Could you check a few things on this model? Use its own coordinates, in mm. Face numbers are marked on the shaded views. Round coordinates to 2 decimals unless told otherwise and drop trailing zeros. Write each loop counter-clockwise with the first axis right and the second up, starting at its lowest first coordinate (ties: lowest second). Pieces come first, ordered by that corner, then holes. Notation, with made-up numbers: (19, 85) -> (51, 85) arc R12 ccw to (51, 92) -> close; hole circle Ø11 at (51, 1). An arc over 180 degrees is marked (long way). Answer in a Markdown table with one row per item.
from build123d import *

# Parameters (mm, degrees)
SKETCH1_W           = 50
SKETCH1_H           = 50
BOSS_EXTRUDE1_DEPTH = 6
CUT_EXTRUDE1_REACH  = 39.336
SKETCH5_R           = 5
CHAMFER1_SIZE       = 1
CHAMFER2_SIZE       = 0.5
M6_TAPPED_HOLE1_D   = 5
SKETCH10_R          = 6.25
CUT_EXTRUDE2_DEPTH  = 2
CIRPATTERN1_COUNT   = 4


# Read off the part's stored shape, not the designer's step: Draft1
with BuildPart() as part:
    # Sketch1 → Boss-Extrude1 (new, symmetric)
    with BuildSketch(Plane.XY):
        Rectangle(SKETCH1_W, SKETCH1_H)
    extrude(amount=BOSS_EXTRUDE1_DEPTH, both=True)

    # Sketch5 → Cut-Extrude1 (cut, up to next)
    with BuildSketch(Plane.XY.offset(6), mode=Mode.PRIVATE) as cut_extrude1_sk1:
        Circle(SKETCH5_R)
    cut_extrude1_tool1 = extrude(cut_extrude1_sk1.sketch, amount=-CUT_EXTRUDE1_REACH, mode=Mode.PRIVATE) & part.part
    add(cut_extrude1_tool1.solids().sort_by_distance((0, 0, 6))[0], mode=Mode.SUBTRACT)

    # Chamfer1
    chamfer1_edges = [part.edges().sort_by_distance(p)[0] for p in [
        (25, -25, 0),
        (-25, -25, 0),
        (-25, 25, 0),
        (25, 25, 0),
    ]]
    chamfer(chamfer1_edges, length=CHAMFER1_SIZE)

    # Chamfer2
    chamfer2_edges = [part.edges().sort_by_distance(p)[0] for p in [
        (0, -25, 6),
        (0, -25, -6),
        (0, 25, -6),
        (0, 25, 6),
        (25, 0, -6),
        (25, 0, 6),
        (-25, 0, -6),
        (-25, 0, 6),
    ]]
    chamfer(chamfer2_edges, length=CHAMFER2_SIZE - 0.0001)  # a hair under: the kernel refuses the full size

    # M6 Tapped Hole1 (through all)
    with Locations(Plane.XY.offset(6)):
        with Locations((-16.5, 0), (0, 16.5), (16.5, 0), (0, -16.5)):
            Hole(M6_TAPPED_HOLE1_D / 2)

    # Sketch10 → Cut-Extrude2 (cut)
    with BuildSketch(Plane.XY.offset(6)):
        with Locations((0, 16.5)):
            Circle(SKETCH10_R)
    cut_extrude2 = extrude(amount=-CUT_EXTRUDE2_DEPTH, mode=Mode.SUBTRACT)

    # CirPattern1: Cut-Extrude2 ×4 about axis
    cirpattern1_axis = Axis((0, 0, 0), (0, 0, 1))
    for i in range(1, CIRPATTERN1_COUNT):
        add(cut_extrude2.rotate(cirpattern1_axis, i * 360 / CIRPATTERN1_COUNT), mode=Mode.SUBTRACT)

    # Draft1 outline → Draft1 (revolve, cut)
    with BuildSketch(Plane.XZ):
        Polygon((5, 6), (5, -2.8), (5.69257502, 6), align=None)
    revolve(axis=Axis((0, 0, 0), (0, 0, 1)), mode=Mode.SUBTRACT)


solid = part.part
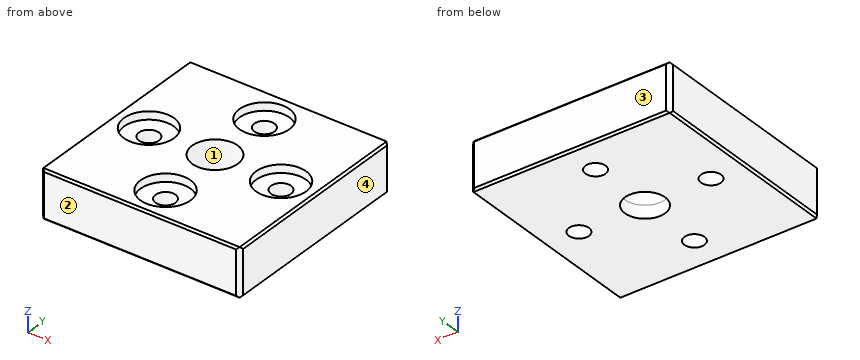
1) Imagine slicing it at D-D, the plane x = 0. Count the separate pieces of the cut face and the enclosed holes in it, plus the area to 3 significant figures.
Findings:
| item | result |
|---|---|
| separate pieces | 4 |
| enclosed holes | 0 |
| area | 323 mm^2 |
2) Imagine slicing it at A-A, the plane x = 16.5. Please give me the cut outline in (y, z), plus the area to 4 significant figures.
Findings:
| item | result |
|---|---|
| outline | (-25, -5.5) -> (-24.5, -6) -> (-2.5, -6) -> (-2.5, 4) -> (-6.25, 4) -> (-6.25, 6) -> (-24.5, 6) -> (-25, 5.5) -> close; (2.5, -6) -> (24.5, -6) -> (25, -5.5) -> (25, 5.5) -> (24.5, 6) -> (6.25, 6) -> (6.25, 4) -> (2.5, 4) -> close |
| area | 524.5 mm^2 |
3) For pin 1 (6 mm diameter, centred on x = -1.5, y = -19.5, fed in from +Z); pin 2 (6 mm diameter, centred on x = -16, y = 1.5, fed in from +Z), each with a flat end and sliding along its axis, tell me the tip position at first contact or that it passes through.
Findings:
| item | result |
|---|---|
| pin 1 | stops at z = 6 |
| pin 2 | stops at z = 4 |
4) Please list where these lines run through material, in increasing order: line 1 (Y direction, x = 0, z = 5.3); line 2 (Y direction, x = 0, z = 1.25); line 3 (Y direction, x = -16.5, z = 4.9).
Findings:
| item | result |
|---|---|
| line 1 | y = -25 to -22.75, -10.25 to -5.64, 5.64 to 10.25, 22.75 to 25 |
| line 2 | y = -25 to -19, -14 to -5.32, 5.32 to 14, 19 to 25 |
| line 3 | y = -25 to -6.25, 6.25 to 25 |
5) Thinking about a two-plate mould opening in Y: for the marked faces 1, 2, 3 and 4, which applies, +Y half, -Y half, draft (parallel to the pull), parting line (faces both ways), or undercut?
Findings:
| item | result |
|---|---|
| face 1 | undercut |
| face 2 | -Y half |
| face 3 | +Y half |
| face 4 | draft |
6) Imagine slicing it at C-C, the plane z = -3.5. Please give me the cut outline in (x, y).
Findings:
| item | result |
|---|---|
| outline | (-25, -24) -> (-24, -25) -> (24, -25) -> (25, -24) -> (25, 24) -> (24, 25) -> (-24, 25) -> (-25, 24) -> close; hole circle Ø5 at (-16.5, 0); hole circle Ø10 at (0, 0); hole circle Ø5 at (0, -16.5); hole circle Ø5 at (0, 16.5); hole circle Ø5 at (16.5, 0) |
